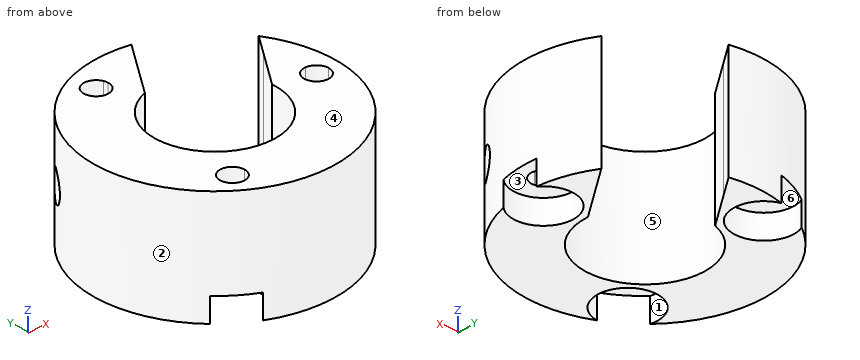
```python
from build123d import *

# Parameters (mm, degrees)
BOSS_EXTRUDE2_DEPTH     = 9.5
CUT_EXTRUDE2_DEPTH      = 27.058535816
CUT_EXTRUDE2_DEPTH_BACK = 27.058535816
SKETCH5_R               = 1.25
SKETCH6_R               = 2.5
CUT_EXTRUDE9_DEPTH      = 2


with BuildPart() as part:
    # Sketch1 → Boss-Extrude2 (new body)
    with BuildSketch(Plane.XY):
        with BuildLine():
            ThreePointArc((-10.902610273, 5.618325714), (-9.358197978, 5.946861897), (-7.779340218, 5.965664362))
            Line((-7.779340218, 5.965664362), (-6.496881129, 7.798486163))
            ThreePointArc((-6.496881129, 7.798486163), (-14.207044336, -10.197524815), (0.057841359, 3.212026405))
            Line((0.057841359, 3.212026405), (-1.224617731, 1.379204604))
            ThreePointArc((-1.224617731, 1.379204604), (-0.701306814, -0.110523909), (-0.480783057, -1.674018275))
            ThreePointArc((-0.480783057, -1.674018275), (0.228827523, -1.982287772), (0.52081643, -2.698751126))
            ThreePointArc((0.52081643, -2.698751126), (0.163849564, -3.476154966), (-0.658416217, -3.71208093))
            ThreePointArc((-0.658416217, -3.71208093), (-5.090643329, -9.253473613), (-12.184684972, -9.091476058))
            ThreePointArc((-12.184684972, -9.091476058), (-13.648069553, -9.398668012), (-13.860882426, -7.918609902))
            ThreePointArc((-13.860882426, -7.918609902), (-16.443755706, -1.309492285), (-12.756440886, 4.753129216))
            ThreePointArc((-12.756440886, 4.753129216), (-12.290784632, 6.174053415), (-10.902610273, 5.618325714))
        make_face()
        with BuildLine():
            ThreePointArc((-3.476685985, -1.839330652), (-11.340506987, -6.10082326), (-10.031408473, 2.747129106))
            Line((-10.031408473, 2.747129106), (-7.779340218, 5.965664362))
            ThreePointArc((-7.779340218, 5.965664362), (-9.358197978, 5.946861897), (-10.902610273, 5.618325714))
            ThreePointArc((-10.902610273, 5.618325714), (-10.850027906, 5.435061947), (-10.832295948, 5.245230202))
            ThreePointArc((-10.832295948, 5.245230202), (-11.60332603, 4.252192297), (-12.756440886, 4.753129216))
            ThreePointArc((-12.756440886, 4.753129216), (-16.443755706, -1.309492285), (-13.860882426, -7.918609902))
            ThreePointArc((-13.860882426, -7.918609902), (-12.721194489, -7.591608608), (-12.035429397, -8.558844193))
            ThreePointArc((-12.035429397, -8.558844193), (-12.073448385, -8.835418744), (-12.184684972, -9.091476058))
            ThreePointArc((-12.184684972, -9.091476058), (-5.090643329, -9.253473613), (-0.658416217, -3.71208093))
            ThreePointArc((-0.658416217, -3.71208093), (-1.52531241, -2.609751731), (-0.480783057, -1.674018275))
            ThreePointArc((-0.480783057, -1.674018275), (-0.701306814, -0.110523909), (-1.224617731, 1.379204604))
            Line((-1.224617731, 1.379204604), (-3.476685985, -1.839330652))
        make_face()
    extrude(amount=BOSS_EXTRUDE2_DEPTH)

    # Sketch5 → Cut-Extrude2 (cut, two sides: drawn at the far end of the back side and taken through both)
    with BuildSketch(Plane(origin=(3.446074086, -2.411281355, 0), x_dir=(0, 0, -1), z_dir=(0.8193403109233307, -0.5733074697717271, 0)).offset(-CUT_EXTRUDE2_DEPTH_BACK)):
        with Locations(Location((-5, -6.500247794, 0), (0, 0, 90))):
            Circle(SKETCH5_R)
    extrude(amount=CUT_EXTRUDE2_DEPTH + CUT_EXTRUDE2_DEPTH_BACK, mode=Mode.SUBTRACT)

    # Sketch6 → Cut-Extrude9 (cut)
    with BuildSketch(Plane(origin=(0, 0, 0), x_dir=(-1, 0, 0), z_dir=(0, 0, -1))):
        with Locations((0.50418357, -2.698751126)):
            Circle(SKETCH6_R)
        with Locations((13.060429397, -8.558844193)):
            Circle(SKETCH6_R)
        with Locations((11.857295948, 5.245230202)):
            Circle(SKETCH6_R)
    extrude(amount=-CUT_EXTRUDE9_DEPTH, mode=Mode.SUBTRACT)


solid = part.part
```
Check sheet for the modelled part. Datum: model origin and axes. Units: mm. Face numbers are marked on the shaded views. A direction names the side the tool comes from. Round coordinates to 2 decimals unless told otherwise and drop trailing zeros. Order: outer loops, then holes, each group sorted by start corner. A loop starts at its lowest first (then second) coordinate and runs counter-clockwise, first axis right, second up. Notation, with made-up numbers: M 54,25 L 76,25 A23 ccw 76,63 Z; hole C 72.5,83 d1. An arc over 180 degrees is marked long. Answer in a Markdown table with one row per item.
(1) Section check D-D on x = -12.5. Give the number of separate pieces and of enclosed holes in the cut face, plus the area to 3 significant figures.
Findings:
| item | result |
|---|---|
| separate pieces | 4 |
| enclosed holes | 0 |
| area | 71.7 mm^2 |
(2) Set-up check for the marked faces 5 and 6: record each of +Z, -Z, +X, -X, +Y, -Y from which the full face is reachable in a straight line by a thin tool's end or side.
Findings:
| item | result |
|---|---|
| face 5 | +Z, -Z |
| face 6 | -Z |
(3) Section check C-C on z = 4.75. Record the boundary of the cut face in (x, y) (3 decimals).
Findings:
| item | result |
|---|---|
| outline | M -17.308,2.682 A10 ccw -1.044,-8.698 L -5.204,-5.787 A5 cw -13.148,-0.228 Z; M -15.904,4.689 L -11.744,1.779 A5 cw -10.031,2.747 L -6.497,7.798 A10 ccw Z; M -3.8,-3.78 L 0.36,-6.691 A10 ccw 0.058,3.212 L -3.477,-1.839 A5 cw Z; hole C -13.06,-8.559 d2.05; hole C -11.857,5.245 d2.05; hole C -0.504,-2.699 d2.05 |
(4) Section check A-A on z = 6.5. Record the boundary of the cut face in (x, y) (3 decimals).
Findings:
| item | result |
|---|---|
| outline | M -10.031,2.747 L -6.497,7.798 A10 ccw long 0.058,3.212 L -3.477,-1.839 A5 cw long Z; hole C -13.06,-8.559 d2.05; hole C -11.857,5.245 d2.05; hole C -0.504,-2.699 d2.05 |
(5) Material ranges on line 1 along Y through (x, z) = (-11.75, 1.5); line 2 along X through (y, z) = (5.5, 5.5); line 3 along X through (y, z) = (6, 5.25), recorded low to high. Write a range as from..to.
Findings:
| item | result |
|---|---|
| line 1 | y = -11.45..-10.69, -6.43..-5.78, 1.77..2.75 |
| line 2 | x = -15.08..-12.85, -10.86..-8.11 |
| line 3 | x = -14.47..-12.55, -11.16..-7.76 |
(6) Section check B-B on x = -8.75. Record the boundary of the cut face in (y, z).
Findings:
| item | result |
|---|---|
| outline | M -12,0 L -7,0 L -7,9.5 L -12,9.5 Z; M 4.58,0 L 7.99,0 L 7.99,9.5 L 4.58,9.5 Z |
(7) Draft check along X on the marked faces 1, 2, 3 and 4. Enter one of: +X half, -X half, draft (parallel to the pull), parting line (faces both ways), or undercut.
Findings:
| item | result |
|---|---|
| face 1 | undercut |
| face 2 | parting line |
| face 3 | undercut |
| face 4 | draft |
(8) Gauge pin test, flat ends, axial feed: pin 1 (5 mm diameter, centred on x = -5, y = 2.5, fed in from +Z); pin 2 (2.5 mm diameter, centred on x = -11.5, y = 5, fed in from -Z); pin 3 (5 mm diameter, centred on y = 1, z = 1.5, fed in from -X). Record the tip position at first contact, or that the pin passes through.
Findings:
| item | result |
|---|---|
| pin 1 | passes through |
| pin 2 | stops at z = 2 |
| pin 3 | stops at x = -18.46 |
